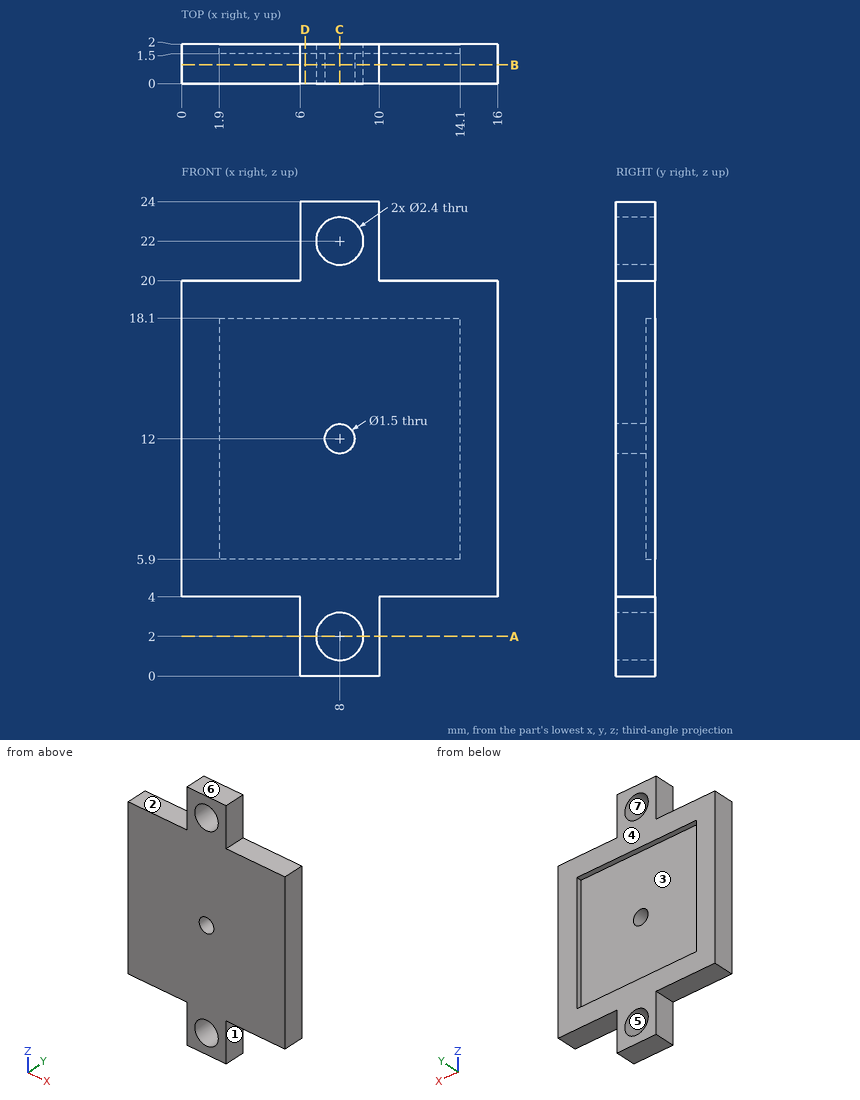
Study the drawing (mm; zero at the part's minimum x, y, z) and answer. A direction names the side the tool comes from. Give positions to 0.01 mm unless a question says otherwise; leave off trailing zeros. Loops run counter-clockwise (first coordinate to the right, second up) from the corner with the lowest first, then second, coordinate; pieces in that order, holes last. Notation, with made-up numbers: (-17, -37.5) -> (11, -37.5) arc R16 ccw to (11, -31.5) -> close; hole circle Ø3 at (-7, 47.25). An arc over 180 degrees is marked (long way). Use a Markdown table: item, result. Add a question column.
1) The part is cut by section A-A, the plane z = 2. Determine the outline of the cut face in (x, y).
2) For a pull along Z with two mould halves and no side action, classify the marked faces 4, 5, 6 and 7 as +Z half, -Z half, draft (parallel to the pull), parting line (faces both ways), or undercut.
3) The part is cut by section B-B, the plane y = 0.95. Determine the outline of the cut face in (x, z).
4) The part is cut by section C-C, the plane x = 8. Determine the outline of the cut face in (y, z), plus the area to 4 significant figures.
5) Each of these flat-tipped pins is pushed along its axis until it touches: P1, Ø0.6, axis at x = 14, y = 1.5, coming from the +Z side; P2, Ø2, axis at x = 8, z = 12, coming from the +Y side; P3, Ø0.6, axis at y = 1.5, z = 22.5, coming from the -X side. Where does it stop, or does it pass through?
6) Consider line 1 along Z through (x, y) = (8, 0.7); line 2 along X through (y, z) = (0.5, 12); line 3 along Z through (x, y) = (13, 1.65). Determine where each line is inside the solid, lowest interval first.
7) Which of the six approach directions +Z, -Z, +X, -X, +Y, -Y give full straight-line access (tool end or side, diameter ignored) to the marked faces 1, 2 and 3?
8) The part is cut by section D-D, the plane x = 6.25. Determine the outline of the cut face in (y, z).
Reported:
| question | item | result |
|---|---|---|
| 1 | outline | (6, 0) -> (6.8, 0) -> (6.8, 2) -> (6, 2) -> close; (9.2, 0) -> (10, 0) -> (10, 2) -> (9.2, 2) -> close |
| 2 | face 4 | draft |
| 2 | face 5 | undercut |
| 2 | face 6 | +Z half |
| 2 | face 7 | undercut |
| 3 | outline | (0, 4) -> (6, 4) -> (6, 0) -> (10, 0) -> (10, 4) -> (16, 4) -> (16, 20) -> (10, 20) -> (10, 24) -> (6, 24) -> (6, 20) -> (0, 20) -> close; hole circle Ø2.4 at (8, 2); hole circle Ø2.4 at (8, 22); hole circle Ø1.5 at (8, 12) |
| 4 | outline | (0, 0) -> (2, 0) -> (2, 0.8) -> (0, 0.8) -> close; (0, 3.2) -> (2, 3.2) -> (2, 5.9) -> (1.5, 5.9) -> (1.5, 11.25) -> (0, 11.25) -> close; (0, 12.75) -> (1.5, 12.75) -> (1.5, 18.1) -> (2, 18.1) -> (2, 20.8) -> (0, 20.8) -> close; (0, 23.2) -> (2, 23.2) -> (2, 24) -> (0, 24) -> close |
| 4 | area | 30.05 mm^2 |
| 5 | P1 | stops at z = 20 |
| 5 | P2 | stops at y = 1.5 |
| 5 | P3 | stops at x = 6 |
| 6 | line 1 | z = 0 to 0.8, 3.2 to 11.25, 12.75 to 20.8, 23.2 to 24 |
| 6 | line 2 | x = 0 to 7.25, 8.75 to 16 |
| 6 | line 3 | z = 4 to 5.9, 18.1 to 20 |
| 7 | face 1 | -Z, +X, +Y, -Y |
| 7 | face 2 | +Z, -X, +Y, -Y |
| 7 | face 3 | +Y |
| 8 | outline | (0, 0) -> (2, 0) -> (2, 5.9) -> (1.5, 5.9) -> (1.5, 18.1) -> (2, 18.1) -> (2, 24) -> (0, 24) -> close |
